Geometry check sheet. Reference: drawing and pictorial views, mm from the part's lowest x, y, z. Give positions to 0.01 mm unless a question says otherwise; leave off trailing zeros. Loops run counter-clockwise (first coordinate to the right, second up) from the corner with the lowest first, then second, coordinate; pieces in that order, holes last. Notation, with made-up numbers: (77, -11.75) -> (131, -11.75) arc R9 cw to (131, -7.75) -> close; hole circle Ø11 at (14.5, 72.25). An arc over 180 degrees is marked (long way). One line per item, written item: value. Start each with the question number.
(1) Sectioned sample at C-C, the plane y = 5.75. Record the cut outline in (x, z).
(2) Sectioned sample at B-B, the plane z = 1.3. Record the cut outline in (x, y).
(3) Scan lines: line 1 along X through (y, z) = (3.75, 1.3); line 2 along Z through (x, y) = (1.3, 0.4). Record each from-to range of solid material in increasing order. Write a range as from..to.
(4) Sectioned sample at D-D, the plane x = 2.4. Record the cut outline in (y, z), then the cut area to 3 significant figures.
(5) Sectioned sample at A-A, the plane x = 1.3. Record the cut outline in (y, z), then the cut area to 3 significant figures.
(6) Draft check along X on the marked faces 1, 2 and 3. Enter one of: pulls with the +X half, pulls with the -X half, needs draft (parallel to the pull), parting line crosses it, or undercut.
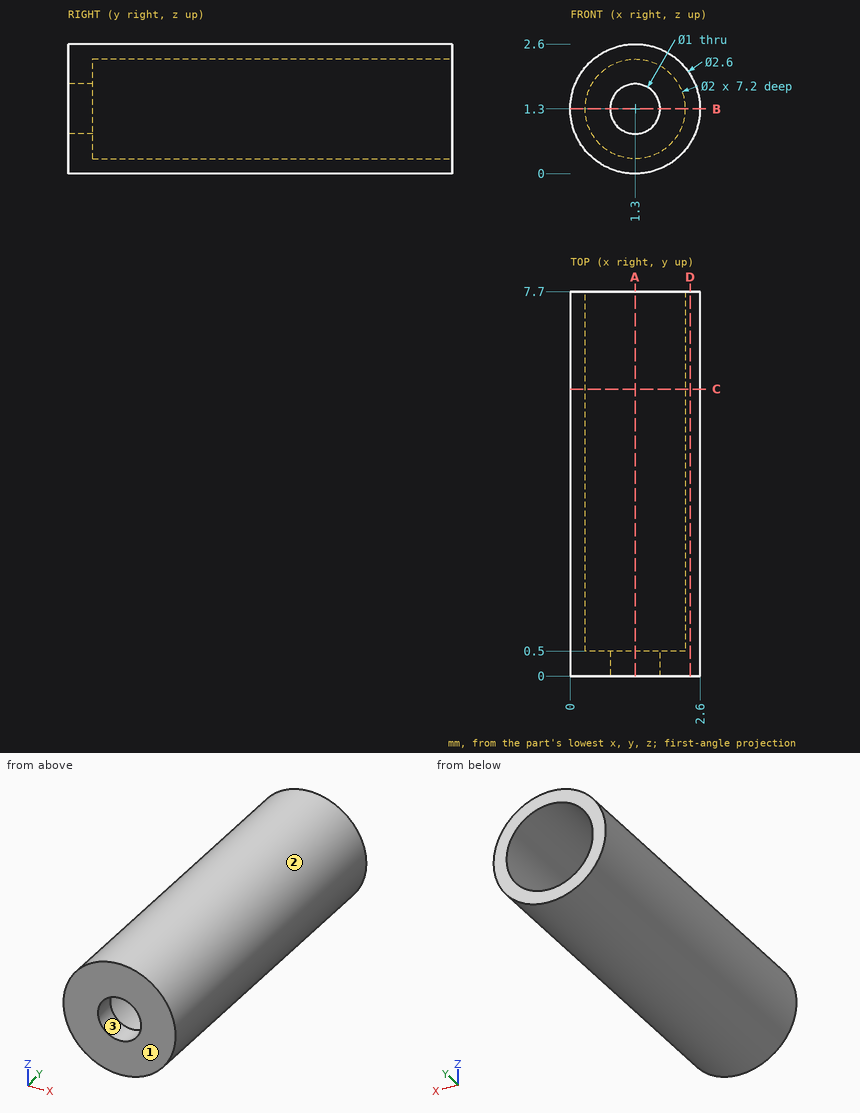
Calculated:
1. outline: circle Ø2.6 at (1.3, 1.3); hole circle Ø2 at (1.3, 1.3)
2. outline: (0, 0) -> (0.8, 0) -> (0.8, 0.5) -> (0.3, 0.5) -> (0.3, 7.7) -> (0, 7.7) -> close; (1.8, 0) -> (2.6, 0) -> (2.6, 7.7) -> (2.3, 7.7) -> (2.3, 0.5) -> (1.8, 0.5) -> close
3. line 1: x = 0..0.3, 2.3..2.6
3. line 2: z = 0..0.8, 1.8..2.6
4. outline: (0, 0.61) -> (7.7, 0.61) -> (7.7, 1.99) -> (0, 1.99) -> close
4. area: 10.7 mm2
5. outline: (0, 0) -> (7.7, 0) -> (7.7, 0.3) -> (0.5, 0.3) -> (0.5, 0.8) -> (0, 0.8) -> close; (0, 1.8) -> (0.5, 1.8) -> (0.5, 2.3) -> (7.7, 2.3) -> (7.7, 2.6) -> (0, 2.6) -> close
5. area: 5.12 mm2
6. face 1: needs draft
6. face 2: parting line crosses it
6. face 3: undercut
